For this review, take the finished solid that the model builds, in its own axes (mm). A direction names the side the tool comes from. Round coordinates to 2 decimals unless told otherwise and drop trailing zeros. Loops run counter-clockwise (first coordinate to the right, second up) from the corner with the lowest first, then second, coordinate; pieces in that order, holes last.
1. Consider section D-D on y = -8.5. State the section outline as (x, z) points, then the cut area to 3 significant figures.
2. Tool access review of faces 1 (the flat face through (-10.4, -9.8, 13.615)), 2 (the flat face through (-14, -26.7, -32)), 3 (the flat face through (-10.4, -9.8, -36.385)), 4 (the flat face through (-10.223, -14.8, -11.7)), 5 (the cylindrical face through (-11.99, 1.37, -30.96)): name each direction out of +Z, -Z, +X, -X, +Y, -Y from which nothing blocks a thin tool from reaching the whole face with its end or side.
3. Consider section B-B on z = -31. State the section outline as (x, y) points.
4. Clearance check with flat-ended pins moving along their axes: pin 1 Ø6 at (y, z) = (-14.5, -2) entering from +X; pin 2 Ø2.5 at (x, z) = (-13, -33) entering from -Y; pin 3 Ø1.6 at (x, z) = (-15, -32) entering from +Y. State where each tip first meets the part, or that it passes through.
5. Consider section C-C on x = -15. State the section outline as (y, z) points, then the cut area to 3 significant figures.
6. Draft analysis for pull direction X (two halves, no side actions). For faces 6 (the flat face through (14.777, 1, -11)), 7 (the cylindrical face through (-11.596, 1.373, 9.27)), 8 (the flat face through (-1, 3, -12)), 9 (the flat face through (-14, -0.3, 10)), state which applies: released by +X, released by -X, zero draft, split by the parting line, or undercut.
7. Consider section A-A on y = -20. State the section outline as (x, z) points.
8. To check wall thickness, follow line 1 along X through (y, z) = (-16, 9); line 2 along Y through (x, z) = (-1, 11.5); line 3 along Y through (x, z) = (-12, -9). State the ranges of each line that lie inside material, in increasing order.
from build123d import *

# Parameters (mm, degrees)
SKETCH1_W           = 25
SKETCH1_H           = 50
SKETCH1_R           = 2.1
BOSS_EXTRUDE1_DEPTH = 3
SKETCH2_W           = 50
SKETCH2_H           = 3
BOSS_EXTRUDE2_DEPTH = 8
SKETCH3_W           = 8
SKETCH3_H           = 50
BOSS_EXTRUDE3_DEPTH = 30
SKETCH4_R           = 2.65
CUT_EXTRUDE1_DEPTH  = 3.3
FILLET1_R           = 1
SKETCH5_R           = 3.868246804
CUT_EXTRUDE2_DEPTH  = 9
FILLET2_R           = 1


with BuildPart() as part:
    # Sketch1 → Boss-Extrude1 (new body)
    with BuildSketch(Plane(origin=(0, 0, 0), x_dir=(1, 0, 0), z_dir=(0, 1, 0))):
        with Locations((2.276951673, 11.384758364)):
            Rectangle(SKETCH1_W, SKETCH1_H)
        with Locations(Location((1.276951673, 11.384758364, 0), (0, 0, 270))):
            Circle(SKETCH1_R, mode=Mode.SUBTRACT)
    extrude(amount=BOSS_EXTRUDE1_DEPTH)

    # Sketch2 → Boss-Extrude2 (add)
    with BuildSketch(Plane.ZY.offset(10.223048327)):
        with Locations((-11.384758364, 1.5)):
            Rectangle(SKETCH2_W, SKETCH2_H)
    extrude(amount=BOSS_EXTRUDE2_DEPTH)

    # Sketch3 → Boss-Extrude3 (add)
    with BuildSketch(Plane.XZ):
        with Locations((-14.223048327, -11.384758364)):
            Rectangle(SKETCH3_W, SKETCH3_H)
    extrude(amount=BOSS_EXTRUDE3_DEPTH)

    # Sketch4 → Cut-Extrude1 (cut)
    with BuildSketch(Plane(origin=(0, 3, 0), x_dir=(1, 0, 0), z_dir=(0, 1, 0))):
        with Locations(Location((-14.223048327, 32.384758364, 0), (0, 0, 270))):
            Circle(SKETCH4_R)
        with Locations(Location((-14.223048327, -9.615241636, 0), (0, 0, 270))):
            Circle(SKETCH4_R)
    cut_extrude1 = extrude(amount=-CUT_EXTRUDE1_DEPTH, mode=Mode.SUBTRACT)

    # Mirror1: Cut-Extrude1 across plane
    add(cut_extrude1.mirror(Plane.ZX.offset(-13.5)), mode=Mode.SUBTRACT)

    # Fillet1
    fillet1_edges = [part.edges().sort_by_distance(p)[0] for p in [
        (1.276951673, 0, -13.484758364),
    ]]
    fillet(fillet1_edges, radius=FILLET1_R)

    # Sketch5 → Cut-Extrude2 (cut)
    with BuildSketch(Plane.ZY.offset(18.223048327)):
        with Locations((-11.836279124, -20)):
            Circle(SKETCH5_R)
    extrude(amount=-CUT_EXTRUDE2_DEPTH, mode=Mode.SUBTRACT)

    # Fillet2
    fillet2_edges = [part.edges().sort_by_distance(p)[0] for p in [
        (-10.223048327, -20, -15.704525928),
    ]]
    fillet(fillet2_edges, radius=FILLET2_R)

    # Mirror2: Cut-Extrude1 across plane
    add(cut_extrude1.mirror(Plane.ZY.offset(1.723048327)), mode=Mode.SUBTRACT)


solid = part.part
Resolved:
1. outline: (-18.22, -36.38) - (-10.22, -36.38) - (-10.22, 13.62) - (-18.22, 13.62) - close
1. area: 400 mm2
2. face 1: +Z, +X, -X, +Y, -Y
2. face 2: -Y
2. face 3: -Z, +X, -X, +Y, -Y
2. face 4: +Z, -Z, +X, -Y
2. face 5: +Y
3. outline: (-18.22, -30) - (-16.48, -30) - (-16.48, -26.7) - (-11.96, -26.7) - (-11.96, -30) - (-10.22, -30) - (-10.22, 0) - (8.52, 0) - (8.52, 3) - (-11.96, 3) - (-11.96, -0.3) - (-16.48, -0.3) - (-16.48, 3) - (-18.22, 3) - close; (13.04, 0) - (14.78, 0) - (14.78, 3) - (13.04, 3) - close
4. pin 1: stops at x = -10.22
4. pin 2: stops at y = -26.7
4. pin 3: stops at y = -0.3
5. outline: (-30, -36.38) - (3, -36.38) - (3, -34.92) - (-0.3, -34.92) - (-0.3, -29.85) - (3, -29.85) - (3, 7.08) - (-0.3, 7.08) - (-0.3, 12.15) - (3, 12.15) - (3, 13.62) - (-30, 13.62) - (-30, 12.15) - (-26.7, 12.15) - (-26.7, 7.08) - (-30, 7.08) - (-30, -29.85) - (-26.7, -29.85) - (-26.7, -34.92) - (-30, -34.92) - close; hole circle Ø7.74 at (-20, -11.84)
5. area: 1,540 mm2
6. face 6: released by +X
6. face 7: undercut
6. face 8: zero draft
6. face 9: undercut
7. outline: (-18.22, -36.38) - (-10.22, -36.38) - (-10.22, -16.7) arc R1 ccw to (-11.22, -15.7) - (-18.22, -15.7) - close; (-18.22, -7.97) - (-11.22, -7.97) arc R1 ccw to (-10.22, -6.97) - (-10.22, 13.62) - (-18.22, 13.62) - close
8. line 1: x = -18.22 to -10.22
8. line 2: y = 0 to 3
8. line 3: y = -30 to -22.63, -17.37 to 3
